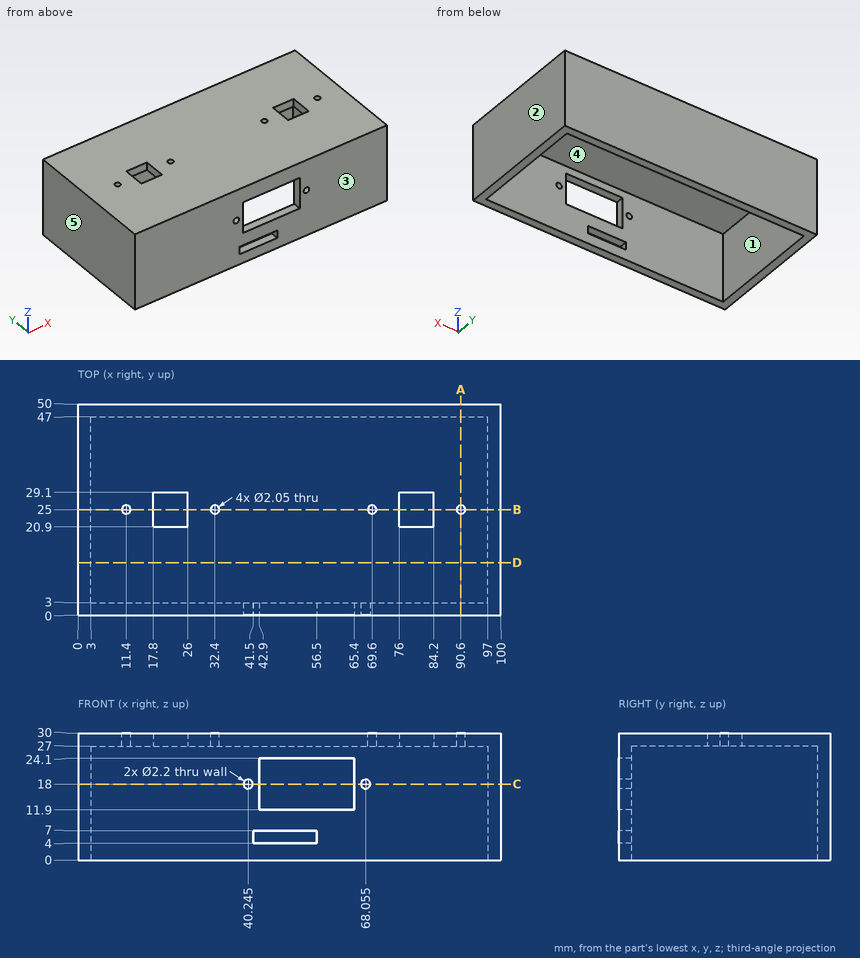
Could you check a few things on this drawing? It's one solid part, dimensions in mm from its lowest x, y, z. A direction names the side the tool comes from. Round coordinates to 2 decimals unless told otherwise and drop trailing zeros. Loops run counter-clockwise (first coordinate to the right, second up) from the corner with the lowest first, then second, coordinate; pieces in that order, holes last. Notation, with made-up numbers: (-33, 86.25) -> (-4, 86.25) arc R29 cw to (-4, 112.25) -> close; hole circle Ø9 at (55.5, 77.5). An arc over 180 degrees is marked (long way). One line per item, written item: value. Start each with the question number.
1. If I drill on probe 1 along X at (y, z) = (22.5, 26.75); probe 2 along Y at (x, z) = (95.5, 8.5); probe 3 along Y at (x, z) = (32.4, 28.1) (3 decimals), over which ranges is the centre line in solid material (lowest first)?
2. For pin 1 (2.5 mm diameter, centred on x = 90.6, y = 25, fed in from -Z), with a flat end and sliding along its axis, tell me the tip position at first contact or that it passes through.
3. If we section it at D-D, the plane y = 12.5: Write out the boundary of the cut face in (x, z).
4. If we mould it in two halves opening along Y, with no side actions, what happens to the marked faces 1, 2 and 3? For each: pulls with the +Y half, pulls with the -Y half, needs draft (parallel to the pull), parting line crosses it, or undercut.
5. For the marked faces 4 and 5, which set-ups out of +Z, -Z, +X, -X, +Y, -Y let a thin tool reach every point of the face, with its end or its side?
6. If we section it at A-A, the plane x = 90.6: Write out the boundary of the cut face in (y, z) (3 decimals), then the cut area to 3 significant figures.
7. If we section it at B-B, the plane y = 25: Give the number of separate pieces and of enclosed holes in the cut face, then the cut area to 3 significant figures.
8. If we section it at C-C, the plane z = 18: Write out the boundary of the cut face in (x, y) (3 decimals), then the cut area to 3 significant figures.
Calculated:
1. probe 1: x = 0 to 3, 97 to 100
1. probe 2: y = 0 to 3, 47 to 50
1. probe 3: y = 0 to 23.975, 26.025 to 50
2. pin 1: stops at z = 27
3. outline: (0, 0) -> (3, 0) -> (3, 27) -> (97, 27) -> (97, 0) -> (100, 0) -> (100, 30) -> (0, 30) -> close
4. face 1: undercut
4. face 2: needs draft
4. face 3: pulls with the -Y half
5. face 4: -Z
5. face 5: +Z, -Z, -X, +Y, -Y
6. outline: (0, 0) -> (3, 0) -> (3, 27) -> (23.975, 27) -> (23.975, 30) -> (0, 30) -> close; (26.025, 27) -> (47, 27) -> (47, 0) -> (50, 0) -> (50, 30) -> (26.025, 30) -> close
6. area: 306 mm²
7. separate pieces: 7
7. enclosed holes: 0
7. area: 388 mm²
8. outline: (0, 0) -> (39.145, 0) -> (39.145, 3) -> (3, 3) -> (3, 47) -> (97, 47) -> (97, 3) -> (69.155, 3) -> (69.155, 0) -> (100, 0) -> (100, 50) -> (0, 50) -> close; (41.345, 0) -> (42.9, 0) -> (42.9, 3) -> (41.345, 3) -> close; (65.4, 0) -> (66.955, 0) -> (66.955, 3) -> (65.4, 3) -> close
8. area: 783 mm²
